Autodesk Inventor part; units mm, degrees
ref_plane "YZ Plane" through (0, 0, 0) normal (1, 0, 0) x (0, 1, 0)
ref_plane "XZ Plane" through (0, 0, 0) normal (0, 1, 0) x (-1, 0, 0)
ref_plane "XY Plane" through (0, 0, 0) normal (0, 0, 1) x (1, 0, 0)
sketch "スケッチ1" plane through (0, 0, 0) normal (0, 0, 1) x (1, 0, 0)
  line L0 (-12.5, 25) -> (12.5, 25)
  line L1 (12.5, 25) -> (12.5, -25)
  line L2 (12.5, -25) -> (-12.5, -25)
  line L3 (-12.5, -25) -> (-12.5, 25)
  line L4 (-10.5, 23) -> (10.5, 23)
  line L5 (10.5, 23) -> (10.5, -23)
  line L6 (10.5, -23) -> (-10.5, -23)
  line L7 (-10.5, -23) -> (-10.5, 23)
  point P0 (0, 0)
  dimension "d0" = 25
  dimension "d1" = 50
  dimension "d2" = 46
  dimension "d3" = 21
  dimension "d4" = 25
  dimension "d5" = 23
  dimension "d6" = 10.5
  dimension "d7" = 12.5
extrude "押し出し1" add sketch "スケッチ1" along normal blind 50
sketch "スケッチ2" plane through (-12.5, 25, 0) normal (0, 1, 0) x (1, 0, 0)
  line L0 (0, 0) -> (25, 0)
  line L1 (0, 0) -> (0, -50)
  arc A0 (6, -33.5) -> (19, -33.5) centre (12.5, -33.5) ccw
  line L2 (6, -33.5) -> (6, 0)
  line L3 (19, -33.5) -> (19, 0)
  point P0 (12.5, 0)
  dimension "d10" = 13
  dimension "d11" = 33.5
  dimension "d12" = 12.5
extrude "押し出し2" cut sketch "スケッチ2" against normal blind 2
sketch "スケッチ3" plane through (-12.5, 25, 50) normal (0, 1, 0) x (1, 0, 0)
  arc A0 (6, 16.5) -> (19, 16.5) centre (12.5, 16.5) ccw
  circle A1 centre (4.5, 10) radius 1.1
  circle A2 centre (4.5, 46) radius 1.1
  circle A3 centre (20.5, 46) radius 1.1
  circle A4 centre (20.5, 10) radius 1.1
  point P0 (12.5, 50)
  dimension "d15" = 6.5
  dimension "d16" = 6.5
  dimension "d17" = 2.2
  dimension "d18" = 8
  dimension "d19" = 8
  dimension "d20" = 8
  dimension "d21" = 8
  dimension "d22" = 29.5
  dimension "d23" = 29.5
hole "穴1" at (-8, 25, 4) at (8, 25, 4) at (8, 25, 40) at (-8, 25, 40) direction (0, -1, 0) diameter 2.2 depth 2 tip angle 118 counterbore diameter 4 counterbore depth 0.5
sketch "スケッチ4" plane through (-12.5, -25, 0) normal (0, -1, 0) x (1, 0, 0)
  line L0 (25, 0) -> (0, 0)
  line L1 (25, 0) -> (25, 50)
  circle A0 centre (12.5, 10.5) radius 2
  point P0 (12.5, 0)
  dimension "d31" = 4
  dimension "d32" = 12.5
  dimension "d33" = 10.5
hole "穴2" at (0, -25, 10.5) direction (0, 1, 0) diameter 4 end through all
sketch "スケッチ5" plane through (-12.5, 25, 50) normal (0, 1, 0) x (1, 0, 0)
  line L0 (0, 0) -> (25, 0)
  arc A0 (6, 16.5) -> (19, 16.5) centre (12.5, 16.5) ccw
  circle A1 centre (20.5, 4) radius 1.5
  circle A2 centre (4.5, 4) radius 1.5
  point P0 (12.5, 50)
  dimension "d43" = 4
  dimension "d44" = 4
  dimension "d46" = 8
  dimension "d47" = 8
  dimension "d57" = 3
hole "穴4" at (-8, 25, 46) at (8, 25, 46) direction (0, -1, 0) diameter 3 end through all
thread "ねじ1"
thread "ねじ2"
thread "ねじ3"
thread "ねじ4"
sketch "スケッチ7" plane through (-12.5, -25, 0) normal (0, -1, 0) x (1, 0, 0)
  line L0 (25, 50) -> (0, 50)
  line L1 (0, 0) -> (0, 50)
  circle A0 centre (12.5, 30) radius 4
  point P0 (12.5, 0)
  dimension "d78" = 8
  dimension "d80" = 20
  dimension "d81" = 12.5
hole "穴5" at (0, -25, 30) direction (0, 1, 0) diameter 8 end through all
properties part number "08" material "アルミニウム 6061"
Part model, mm, in its own coordinate system. A direction names the side the tool comes from. Coordinates: 2 decimals unless noted, no trailing zeros. Loops run counter-clockwise (first coordinate to the right, second up) from the corner with the lowest first, then second, coordinate; pieces in that order, holes last. Notation, with made-up numbers: M 6.25,43.25 L 34.25,43.25 A18 cw 34.25,77.25 Z; hole C -5.75,33 d3. An arc over 180 degrees is marked long. Use a Markdown table: item, result. Add a question column.
Q1. Cut at A-A (x = 0). Write the cut outline in (y, z), and give its area (3 significant figures).
Q2. Pin check, flat tips, straight feed: P1, Ø5, axis at x = 0, z = 10.5, coming from the +Y side; P2, Ø3.5, axis at x = 8, z = 40, coming from the +Y side; P3, Ø2.5, axis at x = 8, z = 46, coming from the +Y side. Stop position of each tip, or through.
Q3. Which spindle directions (+Z, -Z, +X, -X, +Y, -Y) get a long thin tool onto all of the face, cutting with end or side? Do faces 4 (the flat face through (9, 24.5, 3)), 5 (the cylindrical face through (-8.07, 23.99, 44.5)), 6 (the cylindrical face through (0, 24, 40)), 7 (the flat face through (-10.5, 0, 25)). Say none if no direction does.
Q4. Cut at D-D (z = 46). Write the cut outline in (x, y), and give its area (3 significant figures).
Q5. Mould opens along Z. For faces 1 (the cylindrical face through (7.67, 23.74, 41.05)), 2 (the flat face through (-11, 2, 50)), 3 (the flat face through (-12.5, 0, 25)) say: +Z half, -Z half, draft (parallel to the pull), parting line (faces both ways), or undercut.
Q6. Probe L1, parallel to Z at x = 8, y = 24.8; L2, parallel to X at y = -4.5, z = 6; L3, parallel to Y at x = 2.25, z = 41. List the from-to ranges inside material, lowest first.
Q7. Cut at B-B (z = 10.5). Write the cut outline in (x, y), and give its area (3 significant figures).
Q8. Cut at C-C (y = -7.5). Write the cut outline in (x, z).
Worked out:
| question | item | result |
|---|---|---|
| 1 | outline | M -25,0 L -23,0 L -23,8.5 L -25,8.5 Z; M -25,12.5 L -23,12.5 L -23,26 L -25,26 Z; M -25,34 L -23,34 L -23,50 L -25,50 Z; M 23,40 L 25,40 L 25,50 L 23,50 Z |
| 1 | area | 96.0 mm2 |
| 2 | P1 | stops at y = -23 |
| 2 | P2 | stops at y = 24.5 |
| 2 | P3 | passes through |
| 3 | face 4 | +Y |
| 3 | face 5 | +Y, -Y |
| 3 | face 6 | -Z, +Y |
| 3 | face 7 | +Z, -Z |
| 4 | outline | M -12.5,-25 L -9.5,-25 L -9.5,-23 L -10.5,-23 L -10.5,23 L -9.5,23 L -9.5,25 L -12.5,25 Z; M -6.5,-25 L 6.5,-25 L 6.5,-23 L -6.5,-23 Z; M -6.5,23 L 6.5,23 L 6.5,25 L -6.5,25 Z; M 9.5,-25 L 12.5,-25 L 12.5,25 L 9.5,25 L 9.5,23 L 10.5,23 L 10.5,-23 L 9.5,-23 Z |
| 4 | area | 260 mm2 |
| 5 | face 1 | undercut |
| 5 | face 2 | +Z half |
| 5 | face 3 | draft |
| 6 | L1 | z = 0 to 2, 6 to 38, 42 to 44.5, 47.5 to 50 |
| 6 | L2 | x = -12.5 to -10.5, 10.5 to 12.5 |
| 6 | L3 | y = -25 to -23, 23 to 25 |
| 7 | outline | M -12.5,-25 L -2,-25 L -2,-23 L -10.5,-23 L -10.5,23 L -6.5,23 L -6.5,25 L -12.5,25 Z; M 2,-25 L 12.5,-25 L 12.5,25 L 6.5,25 L 6.5,23 L 10.5,23 L 10.5,-23 L 2,-23 Z |
| 7 | area | 250 mm2 |
| 8 | outline | M -12.5,0 L -10.5,0 L -10.5,50 L -12.5,50 Z; M 10.5,0 L 12.5,0 L 12.5,50 L 10.5,50 Z |
